The model under review builds one solid part; all positions refer to its coordinate system, in mm. A direction names the side the tool comes from. Coordinates: 2 decimals unless noted, no trailing zeros. Write each loop counter-clockwise with the first axis right and the second up, starting at its lowest first coordinate (ties: lowest second). Pieces come first, ordered by that corner, then holes. Notation, with made-up numbers: (28, -0.5) - (48, -0.5) arc R23 ccw to (48, 29.5) - close; hole circle Ø6 at (-25.75, 24). An arc over 180 degrees is marked (long way). Use one line per item in the form item = value. Start each with the question number.
```python
from build123d import *

# Parameters (mm, degrees)
F0_W     = 151
F0_H     = 100
F1_DEPTH = 12
F3_DEPTH = 245.5
F5_D     = 12
F5_DEPTH = 12
F5_TIP   = 3.6051637142
F6_W     = 130
F6_H     = 75
F7_DEPTH = 12
F9_D     = 12
F9_DEPTH = 12
F9_TIP   = 3.6051637142


with BuildPart() as f1:
    # F0 (on Top) → F1 (new body)
    with BuildSketch(Plane.XY):
        with Locations((75.5, 50)):
            Rectangle(F0_W, F0_H)
    extrude(amount=F1_DEPTH)

    # F2 (on face) → F3 (join)
    with BuildSketch(Plane(origin=(0, 0, 0), x_dir=(1, 0, 0), z_dir=(0, 0, -1))):
        with BuildLine():
            ThreePointArc((100.9, -30.95), (99.0401280605, -26.4598719395), (94.55, -24.6))
            Line((94.55, -24.6), (56.45, -24.6))
            ThreePointArc((56.45, -24.6), (51.9598719395, -26.4598719395), (50.1, -30.95))
            Line((50.1, -30.95), (50.1, -69.05))
            ThreePointArc((50.1, -69.05), (51.9598719395, -73.5401280605), (56.45, -75.4))
            Line((56.45, -75.4), (94.55, -75.4))
            ThreePointArc((94.55, -75.4), (99.0401280605, -73.5401280605), (100.9, -69.05))
            Line((100.9, -69.05), (100.9, -30.95))
        make_face()
        with BuildLine():
            Line((59.625, -27.775), (91.375, -27.775))
            ThreePointArc((91.375, -27.775), (95.8651280605, -29.6348719395), (97.725, -34.125))
            Line((97.725, -34.125), (97.725, -65.875))
            ThreePointArc((97.725, -65.875), (95.8651280605, -70.3651280605), (91.375, -72.225))
            Line((91.375, -72.225), (59.625, -72.225))
            ThreePointArc((59.625, -72.225), (55.1348719395, -70.3651280605), (53.275, -65.875))
            Line((53.275, -65.875), (53.275, -34.125))
            ThreePointArc((53.275, -34.125), (55.1348719395, -29.6348719395), (59.625, -27.775))
        make_face(mode=Mode.SUBTRACT)
    extrude(amount=F3_DEPTH)

    # F5
    with Locations(Plane.XY.offset(12)):
        with Locations((17.5, 85), (133.5, 85), (133.5, 15), (17.5, 15)):
            Hole(F5_D / 2, depth=F5_DEPTH)
            with Locations((0, 0, -(F5_DEPTH + F5_TIP / 2))):  # 118° drill point
                Cone(0, F5_D / 2, F5_TIP, mode=Mode.SUBTRACT)

    # F6 (on face) → F7 (join)
    with BuildSketch(Plane(origin=(0, 0, -245.5), x_dir=(1, 0, 0), z_dir=(0, 0, -1))):
        with Locations((75.5, -50)):
            Rectangle(F6_W, F6_H)
        with BuildLine():
            ThreePointArc((94.55, -24.6), (99.0401280605, -26.4598719395), (100.9, -30.95))
            Line((100.9, -30.95), (100.9, -69.05))
            ThreePointArc((100.9, -69.05), (99.0401280605, -73.5401280605), (94.55, -75.4))
            Line((94.55, -75.4), (56.45, -75.4))
            ThreePointArc((56.45, -75.4), (51.9598719395, -73.5401280605), (50.1, -69.05))
            Line((50.1, -69.05), (50.1, -30.95))
            ThreePointArc((50.1, -30.95), (51.9598719395, -26.4598719395), (56.45, -24.6))
            Line((56.45, -24.6), (94.55, -24.6))
        make_face(mode=Mode.SUBTRACT)
        with BuildLine():
            Line((100.9, -69.05), (100.9, -30.95))
            ThreePointArc((100.9, -30.95), (99.0401280605, -26.4598719395), (94.55, -24.6))
            Line((94.55, -24.6), (56.45, -24.6))
            ThreePointArc((56.45, -24.6), (51.9598719395, -26.4598719395), (50.1, -30.95))
            Line((50.1, -30.95), (50.1, -69.05))
            ThreePointArc((50.1, -69.05), (51.9598719395, -73.5401280605), (56.45, -75.4))
            Line((56.45, -75.4), (94.55, -75.4))
            ThreePointArc((94.55, -75.4), (99.0401280605, -73.5401280605), (100.9, -69.05))
        make_face()
        with BuildLine():
            Line((53.275, -65.875), (53.275, -34.125))
            ThreePointArc((53.275, -34.125), (55.1348719395, -29.6348719395), (59.625, -27.775))
            Line((59.625, -27.775), (91.375, -27.775))
            ThreePointArc((91.375, -27.775), (95.8651280605, -29.6348719395), (97.725, -34.125))
            Line((97.725, -34.125), (97.725, -65.875))
            ThreePointArc((97.725, -65.875), (95.8651280605, -70.3651280605), (91.375, -72.225))
            Line((91.375, -72.225), (59.625, -72.225))
            ThreePointArc((59.625, -72.225), (55.1348719395, -70.3651280605), (53.275, -65.875))
        make_face(mode=Mode.SUBTRACT)
        with BuildLine():
            ThreePointArc((59.625, -27.775), (55.1348719395, -29.6348719395), (53.275, -34.125))
            Line((53.275, -34.125), (53.275, -65.875))
            ThreePointArc((53.275, -65.875), (55.1348719395, -70.3651280605), (59.625, -72.225))
            Line((59.625, -72.225), (91.375, -72.225))
            ThreePointArc((91.375, -72.225), (95.8651280605, -70.3651280605), (97.725, -65.875))
            Line((97.725, -65.875), (97.725, -34.125))
            ThreePointArc((97.725, -34.125), (95.8651280605, -29.6348719395), (91.375, -27.775))
            Line((91.375, -27.775), (59.625, -27.775))
        make_face()
    extrude(amount=F7_DEPTH)

    # F9
    with Locations(Plane(origin=(0, 0, -257.5), x_dir=(1, 0, 0), z_dir=(0, 0, -1))):
        with Locations((25.5, -27.5), (25.5, -72.5), (125.5, -72.5), (125.5, -27.5)):
            Hole(F9_D / 2, depth=F9_DEPTH)
            with Locations((0, 0, -(F9_DEPTH + F9_TIP / 2))):  # 118° drill point
                Cone(0, F9_D / 2, F9_TIP, mode=Mode.SUBTRACT)


solid = f1.part
```
1. The part is to be moulded in two halves that separate along Z. For faces 1 (the cylindrical face through (55.18, 70.41, -121.03)), 2 (the flat face through (75, 75.4, -121)), 3 (the cylindrical face through (22.26, 11.35, 5.92)), 4 (the flat face through (74, 51, 12)), say which applies: released by +Z, released by -Z, zero draft, split by the parting line, or undercut.
2. Take a section at C-C (x = 79.5). State the section outline as (y, z) points (3 decimals), plus the area to 3 significant figures.
3. For L1, parallel to Y at x = 25.5, z = -248.75; L2, parallel to X at y = 27.5, z = -255; L3, parallel to X at y = 15, z = 6, list the stretches that pass through material, from the lowest coordinate up.
4. Take a section at A-A (x = 36.5). State the section outline as (y, z) points.
5. Take a section at B-B (y = 51.5). State the section outline as (x, z) points (3 decimals).
6. For P1, Ø10, axis at y = 73.5, z = -28.5, coming from the +X side; P2, Ø1.5, axis at y = 64, z = -78, coming from the -X side; P3, Ø7, axis at x = 133.5, y = 85, coming from the +Z side; P4, Ø6, axis at y = 20.5, z = -84.5, coming from the -X side, all flat-tipped, find the tip position at first contact; note any pin that passes through.
7. For faces 5 (the cylindrical face through (52.01, 26.41, -121.03)), 6 (the cylindrical face through (99.09, 26.51, -121.03)), 7 (the cylindrical face through (51.91, 73.49, -121.03)), list the 3-axis set-ups (+Z, -Z, +X, -X, +Y, -Y) from which the entire face can be reached by the end or side of a thin tool; tool diameter is ignored.
Returned:
q1.face_1 = undercut
q1.face_2 = undercut
q1.face_3 = zero draft
q1.face_4 = released by +Z
q2.outline = (0, 0) - (24.6, 0) - (24.6, -245.5) - (12.5, -245.5) - (12.5, -257.5) - (87.5, -257.5) - (87.5, -245.5) - (75.4, -245.5) - (75.4, 0) - (100, 0) - (100, 12) - (0, 12) - close; hole (27.775, -245.5) - (72.225, -245.5) - (72.225, 0) - (27.775, 0) - close
q2.area = 3,660 mm²
q3.L1 = 12.5 to 21.5, 33.5 to 66.5, 78.5 to 87.5
q3.L2 = 10.5 to 19.5, 31.5 to 119.5, 131.5 to 140.5
q3.L3 = 0 to 11.5, 23.5 to 127.5, 139.5 to 151
q4.outline = (0, 0) - (100, 0) - (100, 12) - (0, 12) - close; (12.5, -257.5) - (87.5, -257.5) - (87.5, -245.5) - (12.5, -245.5) - close
q5.outline = (0, 0) - (50.1, 0) - (50.1, -245.5) - (10.5, -245.5) - (10.5, -257.5) - (140.5, -257.5) - (140.5, -245.5) - (100.9, -245.5) - (100.9, 0) - (151, 0) - (151, 12) - (0, 12) - close; hole (53.275, -245.5) - (97.725, -245.5) - (97.725, 0) - (53.275, 0) - close
q6.P1 = 100.9
q6.P2 = 50.1
q6.P3 = -245.5
q6.P4 = through
q7.face_5 = -X, -Y
q7.face_6 = +X, -Y
q7.face_7 = -X, +Y
